Check sheet for the drawn part. Datum: minimum x, y, z corner. Units: mm. A direction names the side the tool comes from. Give positions to 0.01 mm unless a question says otherwise; leave off trailing zeros. Loops run counter-clockwise (first coordinate to the right, second up) from the corner with the lowest first, then second, coordinate; pieces in that order, holes last. Notation, with made-up numbers: (89.5, -17) - (141.5, -17) arc R31 cw to (141.5, 18) - close; hole circle Ø4 at (-21.75, 9.5). An arc over 180 degrees is marked (long way). One line per item, written item: value. Start each with the question number.
1. Sectioned sample at A-A (x = 21.25). Record the cut outline in (y, z) (3 decimals), plus the area to 3 significant figures.
2. Mould release check, pull along X, two halves, no side actions. Record for the marked faces 4, 5 and 6: pulls with the +X half, pulls with the -X half, needs draft (parallel to the pull), parting line crosses it, or undercut.
3. Sectioned sample at D-D (y = 13). Record the cut outline in (x, z).
4. Access from +Z, -Z, +X, -X, +Y, -Y to the whole of each face (thin tool, end or side, straight path). Record for the marked faces 1, 2 and 3.
5. Sectioned sample at B-B (y = 3). Record the cut outline in (x, z) (3 decimals).
6. Sectioned sample at C-C (x = 3.25). Record the cut outline in (y, z) (3 decimals), plus the area to 3 significant figures.
7. Gauge pin test, flat ends, axial feed: pin 1 (1.6 mm diameter, centred on x = 5.5, z = 1, fed in from +Y); pin 2 (1.6 mm diameter, centred on x = 19.5, z = 1.5, fed in from +Y); pin 3 (1.6 mm diameter, centred on y = 5.5, z = 2, fed in from +X). Record the tip position at first contact, or that the pin passes through.
8. Scan lines: L1, parallel to X at y = 11.5, z = 3; L2, parallel to X at y = 5, z = 2.8 (3 decimals); L3, parallel to Y at x = 4.5, z = 1.5 (3 decimals). Record each from-to range of solid material in increasing order. Write a range as [from, to].
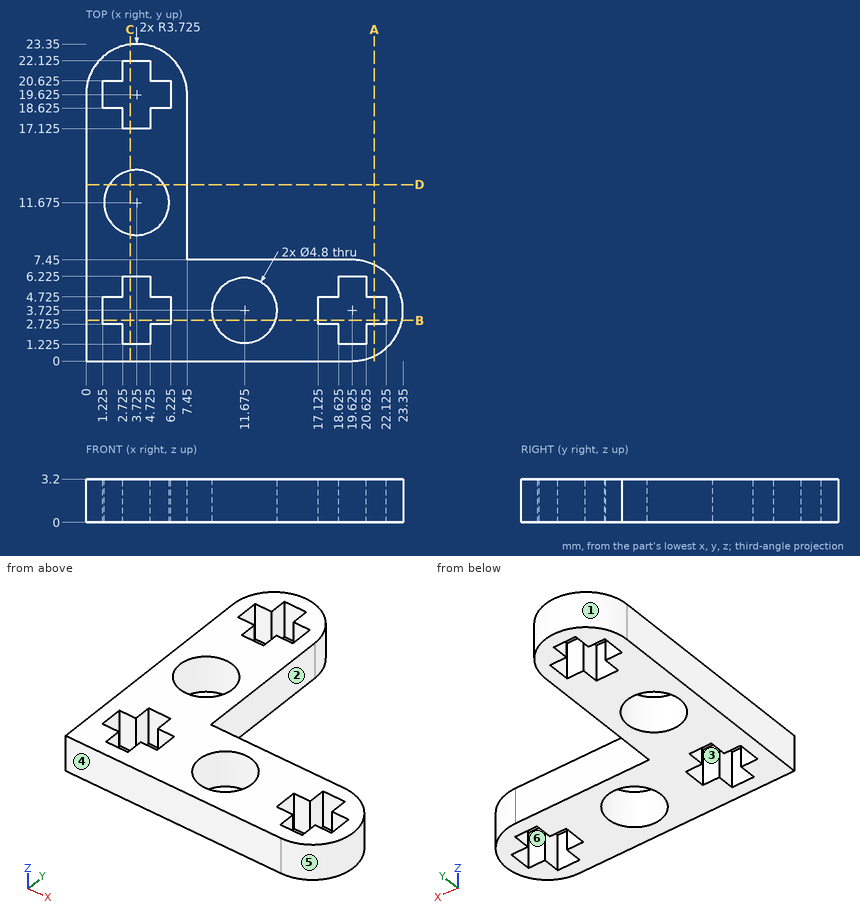
Results are:
1. outline: (0.373, 0) - (2.725, 0) - (2.725, 3.2) - (0.373, 3.2) - close; (4.725, 0) - (7.077, 0) - (7.077, 3.2) - (4.725, 3.2) - close
1. area: 15.1 mm^2
2. face 4: needs draft
2. face 5: pulls with the +X half
2. face 6: undercut
3. outline: (0, 0) - (1.72, 0) - (1.72, 3.2) - (0, 3.2) - close; (5.73, 0) - (7.45, 0) - (7.45, 3.2) - (5.73, 3.2) - close
4. face 1: +Z, -Z, +Y
4. face 2: +Z, -Z, +X, +Y
4. face 3: +Z, -Z
5. outline: (0, 0) - (1.225, 0) - (1.225, 3.2) - (0, 3.2) - close; (6.225, 0) - (9.387, 0) - (9.387, 3.2) - (6.225, 3.2) - close; (13.963, 0) - (17.125, 0) - (17.125, 3.2) - (13.963, 3.2) - close; (22.125, 0) - (23.279, 0) - (23.279, 3.2) - (22.125, 3.2) - close
6. outline: (0, 0) - (1.225, 0) - (1.225, 3.2) - (0, 3.2) - close; (6.225, 0) - (9.322, 0) - (9.322, 3.2) - (6.225, 3.2) - close; (14.028, 0) - (17.125, 0) - (17.125, 3.2) - (14.028, 3.2) - close; (22.125, 0) - (23.32, 0) - (23.32, 3.2) - (22.125, 3.2) - close
6. area: 27.6 mm^2
7. pin 1: stops at y = 23.22
7. pin 2: stops at y = 7.45
7. pin 3: stops at x = 23.22
8. L1: x = [0, 1.33], [6.12, 7.45]
8. L2: x = [0, 2.725], [4.725, 9.642], [13.708, 18.625], [20.625, 23.125]
8. L3: y = [0, 1.225], [6.225, 9.404], [13.946, 17.125], [22.125, 23.268]
